from build123d import *

# Parameters (mm, degrees)
SKETCH_1_R          = 15
EXTRUDE_1_DEPTH     = 7
SKETCH_2_W          = 5.5
SKETCH_2_H          = 3.5
CUT_EXTRUDE_1_DEPTH = 23.338307904
SKETCH_3_R          = 37.5
SKETCH_3_R_2        = 10.340446081
EXTRUDE_2_DEPTH     = 2


with BuildPart() as part:
    # 草图1 → 凸台-拉伸1 (new body)
    with BuildSketch(Plane(origin=(0, 0, 0), x_dir=(1, 0, 0), z_dir=(0, 1, 0))):
        with Locations(Location((0, 0, 0), (0, 0, 270))):
            Circle(SKETCH_1_R)
    extrude(amount=EXTRUDE_1_DEPTH)

    # 草图2 → 切除-拉伸1 (cut, through all)
    with BuildSketch(Plane(origin=(0, 7, 0), x_dir=(1, 0, 0), z_dir=(0, 1, 0))):
        Rectangle(SKETCH_2_W, SKETCH_2_H)
    extrude(amount=-CUT_EXTRUDE_1_DEPTH, mode=Mode.SUBTRACT)

    # 草图3 → 凸台-拉伸2 (add)
    with BuildSketch(Plane.XZ):
        with Locations(Location((0, 0, 0), (0, 0, 270))):
            Circle(SKETCH_3_R)
        Circle(SKETCH_3_R_2, mode=Mode.SUBTRACT)
    extrude(amount=-EXTRUDE_2_DEPTH)


solid = part.part
Could you check a few things on this model? Use its own coordinates, in mm. A direction names the side the tool comes from. Round coordinates to 2 decimals unless told otherwise and drop trailing zeros. Order: outer loops, then holes, each group sorted by start corner. A loop starts at its lowest first (then second) coordinate and runs counter-clockwise, first axis right, second up. Notation, with made-up numbers: M -6,73 L 20,73 A34 ccw 20,108 Z; hole C -35,-2.5 d11. An arc over 180 degrees is marked long. One line per item, written item: value.
(1) Imagine slicing it at A-A (x = 0). Write out the boundary of the cut face in (y, z), and give its area (4 significant figures).
Ans:
outline: M 0,-37.5 L 2,-37.5 L 2,-15 L 7,-15 L 7,-1.75 L 0,-1.75 Z; M 0,1.75 L 7,1.75 L 7,15 L 2,15 L 2,37.5 L 0,37.5 Z
area: 275.5 mm^2
(2) If we mould it in two halves opening along X, with no side actions, what happens to faces 1 (the flat face through (-8, 0, 1)), 2 (the flat face through (-2.75, 4, 0)), 3 (the cylindrical face through (-22.818, 0.986, 29.759))? For each: released by +X, released by -X, zero draft, split by the parting line, or undercut.
Ans:
face 1: zero draft
face 2: undercut
face 3: split by the parting line
(3) I'm going to push flat-ended pins straight in: P1, Ø2, axis at x = -21, z = -3.5, coming from the +Y side; P2, Ø1, axis at x = 3.5, y = 1.5, coming from the -Z side; P3, Ø3, axis at y = 4, z = -0.5, coming from the -X side. Where does each tip first touch, or does it pass through?
Ans:
P1: stops at y = 2
P2: stops at z = -37.38
P3: stops at x = -15
(4) Which directions (+Z, -Z, +X, -X, +Y, -Y) give clear straight access to the entire face, cutting with the end or side of a thin tool? Please do faces 4 (the flat face through (0, 4, 1.75)), 5 (the flat face through (0, 7, 3)), 6 (the flat face through (-16, 2, 1)).
Ans:
face 4: +Y, -Y
face 5: +Z, -Z, +X, -X, +Y
face 6: +Y
(5) Imagine slicing it at B-B (z = 0). Write out the boundary of the cut face in (x, y), and give its area (4 significant figures).
Ans:
outline: M -37.5,0 L -2.75,0 L -2.75,7 L -15,7 L -15,2 L -37.5,2 Z; M 2.75,0 L 37.5,0 L 37.5,2 L 15,2 L 15,7 L 2.75,7 Z
area: 261.5 mm^2
(6) Imagine slicing it at D-D (z = 19). Write out the boundary of the cut face in (x, y), and give its area (3 significant figures).
Ans:
outline: M -32.33,0 L 32.33,0 L 32.33,2 L -32.33,2 Z
area: 129 mm^2
(7) Imagine slicing it at C-C (y = 3). Write out the boundary of the cut face in (x, z).
Ans:
outline: C 0,0 d30; hole M -2.75,-1.75 L 2.75,-1.75 L 2.75,1.75 L -2.75,1.75 Z
(8) I need wall thicknesses on line 1 along Y through (x, z) = (15.5, -5); line 2 along Z through (x, y) = (0.5, 0.5); line 3 along X through (y, z) = (0.75, 23.5). Which ranges of each line are inside material? Lowest first, please. Write a range as from..to.
Ans:
line 1: y = 0..2
line 2: z = -37.5..-1.75, 1.75..37.5
line 3: x = -29.22..29.22
